Build history of the part. All positions in model axes, mm. Round coordinates to 2 decimals unless told otherwise and drop trailing zeros. Loops run counter-clockwise (first coordinate to the right, second up) from the corner with the lowest first, then second, coordinate; pieces in that order, holes last. Notation, with made-up numbers: (62.25, -19) - (72.25, -19) arc R21 cw to (72.25, 16) - close; hole circle Ø5 at (20.25, -24.5). An arc over 180 degrees is marked (long way). Use one line per item in the form item = value. Start each with the question number.
Q1. Pin check, flat tips, straight feed: pin 1 (10 mm diameter, centred on y = 2.5, z = -15.5, fed in from -X); pin 2 (1 mm diameter, centred on x = 2.5, z = -9.5, fed in from -Y). Stop position of each tip, or through.
Q2. Saw through at D-D (y = 9.5). Give the cut face in (x, z), then the cut area to 3 significant figures.
Q3. Drill centre lines: line 1 (Z direction, x = 0, y = 14.4); line 2 (Y direction, x = -2.75, z = -30.5); line 3 (Z direction, x = -1, y = 4). Where is each one in solid material? Low to high.
Q4. Mould opens along X. For faces 1 (the face through (0, 0, 2)), 2 (the face through (4.85, 14, -18)), 3 (the face through (-4.85, 14, -17)), 4 (the face through (-0.06, 14.04, -36.85)) say: released by +X, released by -X, zero draft, split by the parting line, or undercut.
Q5. Saw through at A-A (y = 13). Give the cut face in (x, z), then the cut area to 3 significant figures.
Q6. Saw through at C-C (x = -4). Give the cut face in (y, z).
Q7. Saw through at B-B (z = -34). Give the cut face in (x, y).
```python
from build123d import *
from build123d.topology import SkipClean

# Parameters (mm, degrees)
SKETCH1_R           = 4.85
SKETCH1_R_2         = 1.5
BOSS_EXTRUDE1_DEPTH = 11
BOSS_EXTRUDE2_DEPTH = 6
SKETCH3_R           = 2
CUT_EXTRUDE1_DEPTH  = 7
SKETCH6_R           = 1.5
CUT_EXTRUDE2_DEPTH  = 10


with BuildPart() as part:
    # Sketch1 → Boss-Extrude1 (new body)
    with BuildSketch(Plane(origin=(0, 0, 0), x_dir=(1, 0, 0), z_dir=(0, 1, 0))):
        with Locations(Location((0, 0, 0), (0, 0, 270))):
            Circle(SKETCH1_R)
        with Locations(Location((0, 0, 0), (0, 0, 270))):
            Circle(SKETCH1_R_2, mode=Mode.SUBTRACT)
    extrude(amount=BOSS_EXTRUDE1_DEPTH)

    # Sketch2 → Boss-Extrude2 (add)
    with SkipClean():  # the faces are left unmerged after this step: merging them gives an invalid solid
        with BuildSketch(Plane(origin=(0, 11, 0), x_dir=(1, 0, 0), z_dir=(0, 1, 0))):
            with BuildLine():
                Line((-4.85, 0), (-4.85, 35))
                ThreePointArc((-4.85, 35), (0, 39.85), (4.85, 35))
                Line((4.85, 35), (4.85, 0))
                ThreePointArc((4.85, 0), (0, -4.85), (-4.85, 0))
            make_face()
        extrude(amount=BOSS_EXTRUDE2_DEPTH)
    add(part.part.scale(1), mode=Mode.REPLACE)  # the faces are merged on a copy

    # Sketch3 → Cut-Extrude1 (cut)
    with BuildSketch(Plane(origin=(0, 17, 0), x_dir=(1, 0, 0), z_dir=(0, 1, 0))):
        with Locations(Location((-0.15, 34.852250506, 0), (0, 0, 270))):
            Circle(SKETCH3_R)
    extrude(amount=-CUT_EXTRUDE1_DEPTH, mode=Mode.SUBTRACT)

    # Sketch6 → Cut-Extrude2 (cut)
    with BuildSketch(Plane.XZ.offset(-11)):
        with Locations(Location((0, 0, 0), (0, 0, 90))):
            Circle(SKETCH6_R)
    extrude(amount=-CUT_EXTRUDE2_DEPTH, mode=Mode.SUBTRACT)


solid = part.part
```
Report:
q1.pin_1 = through
q1.pin_2 = 11
q2.outline = circle Ø9.7 at (0, 0); hole circle Ø3 at (0, 0)
q2.area = 66.8 mm²
q3.line_1 = -39.85 to -36.85, -32.86 to -1.5, 1.5 to 4.85
q3.line_2 = 11 to 17
q3.line_3 = -4.75 to -1.12, 1.12 to 4.75
q4.face_1 = zero draft
q4.face_2 = released by +X
q4.face_3 = released by -X
q4.face_4 = undercut
q5.outline = (-4.85, -35) arc R4.85 ccw to (4.85, -35) - (4.85, 0) arc R4.85 ccw to (-4.85, 0) - close; hole circle Ø4 at (-0.15, -34.85); hole circle Ø3 at (0, 0)
q5.area = 394 mm²
q6.outline = (0, -2.74) - (11, -2.74) - (11, -37.74) - (17, -37.74) - (17, 2.74) - (0, 2.74) - close
q7.outline = (-4.85, 11) - (-1.96, 11) - (-1.96, 17) - (-4.85, 17) - close; (1.66, 11) - (4.85, 11) - (4.85, 17) - (1.66, 17) - close
